The listing builds one solid part. Answer for the finished solid, in the listing's coordinates (mm). Face numbers are marked on the shaded views. Round coordinates to 2 decimals unless told otherwise and drop trailing zeros. Write each loop counter-clockwise with the first axis right and the second up, starting at its lowest first coordinate (ties: lowest second). Pieces come first, ordered by that corner, then holes. Notation, with made-up numbers: M 10.5,51 L 56.5,51 A17 ccw 56.5,83 Z; hole C 25.25,-3 d3. An arc over 180 degrees is marked long. Put each result on its own line as item: value. Start each with the question number.
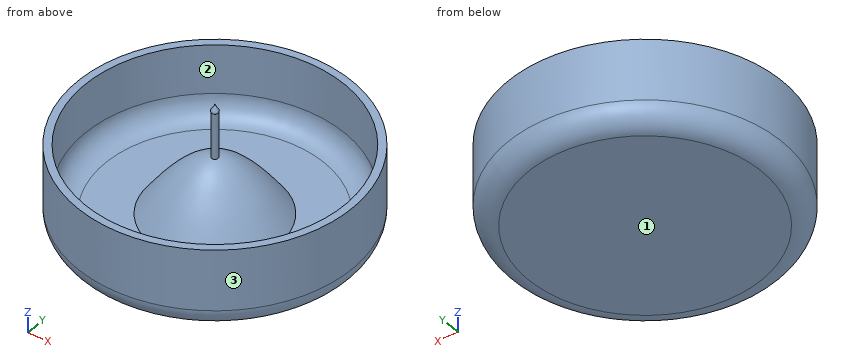
```python
from build123d import *

# Parameters (mm, degrees)
F0_R     = 42.672
F0_R_2   = 40.386
F2_DEPTH = 25.4
F3_DEPTH = 3.81
F5_R     = 6.35


# Not quite as in the source:
# - a feature names something its author has since deleted; it is built from what else it names


with BuildPart() as f2:
    # F0 (on Top) → F2 (new body)
    with BuildSketch(Plane.XY):
        Circle(F0_R)
        Circle(F0_R_2, mode=Mode.SUBTRACT)
    extrude(amount=F2_DEPTH)

    # F0 (on Top) → F3 (join)
    with BuildSketch(Plane.XY):
        Circle(F0_R_2)
    extrude(amount=F3_DEPTH)

    # F1 (on Front) → F4 (revolve)
    with BuildSketch(Plane.XZ):
        with BuildLine():
            Line((-22.661603124, 0), (-0.3999708066, 0))
            Line((-0.3999708066, 0), (0, 0))
            Line((0, 0), (0, 21.5927247815))
            add(Edge.make_bspline(
                [(-0.9605343803, 21.5162747094), (-0.7741159133, 21.5404865376), (-0.4544785974, 21.5726982013), (-0.1335448781, 21.5887811226), (0, 21.5927247815)],
                knots=[0.4844452831, 0.4844452831, 0.4844452831, 0.4844452831, 0.4961290643, 0.5044321792, 0.5044321792, 0.5044321792, 0.5044321792], degree=3))
            add(Edge.make_bspline(
                [(-22.661603124, 0), (-15.6758083409, 10.256190155), (-8.6900138326, 20.5123783076), (-0.9605343803, 21.5162747094)],
                knots=[0, 0, 0, 0, 0.4844452831, 0.4844452831, 0.4844452831, 0.4844452831], degree=3))
        make_face()
        with BuildLine():
            Line((-0.9605343803, 35.6623469879), (0, 35.6623469879))
            Line((0, 35.6623469879), (0, 38.5057479143))
            add(Edge.make_bspline(
                [(0, 38.5057479143), (0, 37.0840474511), (-1.5196733875, 36.4921689034), (-0.9605343803, 35.6623469879)],
                knots=[0, 0, 0, 0, 3.0012589232, 3.0012589232, 3.0012589232, 3.0012589232], degree=3))
        make_face()
        with BuildLine():
            add(Edge.make_bspline(
                [(-0.9605343803, 21.5162747094), (-0.7741159133, 21.5404865376), (-0.4544785974, 21.5726982013), (-0.1335448781, 21.5887811226), (0, 21.5927247815)],
                knots=[0.4844452831, 0.4844452831, 0.4844452831, 0.4844452831, 0.4961290643, 0.5044321792, 0.5044321792, 0.5044321792, 0.5044321792], degree=3))
            Line((0, 21.5927247815), (0, 35.6623469879))
            Line((0, 35.6623469879), (-0.9605343803, 35.6623469879))
            Line((-0.9605343803, 35.6623469879), (-0.9605343803, 21.5162747094))
        make_face()
    revolve(axis=Axis((0, 0, 17.8311734939), (0, 0, -1)))

    # F5
    f5_edges = [f2.edges().sort_by_distance(p)[0] for p in [
        (-40.386, 0, 3.81),
        (-42.672, 0, 0),
    ]]
    fillet(f5_edges, radius=F5_R)


solid = f2.part
```
Item 1: Flat-ended cylindrical pins translate along their axes: pin 1 (3 mm diameter, centred on x = 17.5, y = -33, fed in from +Z); pin 2 (12 mm diameter, centred on x = -31, z = 10, fed in from -Y); pin 3 (12 mm diameter, centred on y = 14, z = 19.5, fed in from -X). Find the tip coordinate at first contact, or state that the pin passes through.
Item 2: Section B-B (z = 28) is taken. Give the vertices of the cut face in (x, y), and give its area (3 significant figures).
Item 3: Section A-A (z = 23.5) is taken. Give the vertices of the cut face in (x, y).
Item 4: Section C-C (z = 16) is taken. Count the separate pieces of the cut face and the enclosed holes in it, and give its area (3 significant figures).
Item 5: Determine the mould class of the marked faces 1, 2 and 3 for opening direction X: released by +X, released by -X, zero draft, split by the parting line, or undercut.
Item 6: Consider line 1 along Y through (x, z) = (0, 22); line 2 along X through (y, z) = (-0.5, 13.5); line 3 along Y through (x, z) = (0, 19.25). Determine where each line is inside the solid, lowest interval first. Write a range as [from, to].
Output values:
1. pin 1: stops at z = 6.02
1. pin 2: stops at y = -34.58
1. pin 3: stops at x = -41.92
2. outline: C 0,0 d1.92
2. area: 2.90 mm^2
3. outline: C 0,0 d85.34; C 0,0 d1.92; hole C 0,0 d80.77
4. separate pieces: 2
4. enclosed holes: 1
4. area: 936 mm^2
5. face 1: zero draft
5. face 2: undercut
5. face 3: split by the parting line
6. line 1: y = [-42.67, -40.39], [-0.96, 0.96], [40.39, 42.67]
6. line 2: x = [-42.67, -40.38], [-12.73, 12.73], [40.38, 42.67]
6. line 3: y = [-42.67, -40.39], [-6.52, 6.52], [40.39, 42.67]
